Work out the finished part from the listing and answer in its coordinate system (mm). Face numbers are marked on the shaded views. A direction names the side the tool comes from. Round coordinates to 2 decimals unless told otherwise and drop trailing zeros. Loops run counter-clockwise (first coordinate to the right, second up) from the corner with the lowest first, then second, coordinate; pieces in that order, holes last. Notation, with made-up numbers: (-37, 85) -> (-22, 85) arc R25 ccw to (-22, 104) -> close; hole circle Ø4 at (-36.5, -26). An arc over 180 degrees is marked (long way). Use one line per item in the form item = value.
```python
from build123d import *

# Parameters (mm, degrees)
F1_DEPTH = 12.7
F3_DEPTH = 38.1
F4_W     = 38.1
F4_H     = 12.7
F5_DEPTH = 50.801
F7_DEPTH = 76.201


with BuildPart() as f1:
    # F0 (on Front) → F1 (new body)
    with BuildSketch(Plane.XZ):
        Polygon((0, 25.4), (0, 0), (76.2, 0), (76.2, 25.4), (50.8, 50.8), (25.4, 50.8), align=None)
    extrude(amount=F1_DEPTH)

    # F2 (on face) → F3 (join)
    with BuildSketch(Plane.XZ.offset(12.7)):
        Polygon((38.1, 50.8), (0, 0), (76.2, 0), align=None)
    extrude(amount=F3_DEPTH)

    # F4 (on face) → F5 (cut, through all)
    with BuildSketch(Plane(origin=(0, 0, 0), x_dir=(-1, 0, 0), z_dir=(0, 1, 0))):
        with Locations((-38.1, 6.35)):
            Rectangle(F4_W, F4_H)
    extrude(amount=-F5_DEPTH, mode=Mode.SUBTRACT)

    # F6 (on face) → F7 (cut, through all)
    with BuildSketch(Plane.YZ.offset(76.2)):
        Polygon((-12.7, 38.1), (-12.7, 50.8), (-50.8, 50.8), (-50.8, 0), align=None)
    extrude(amount=-F7_DEPTH, mode=Mode.SUBTRACT)


solid = f1.part
```
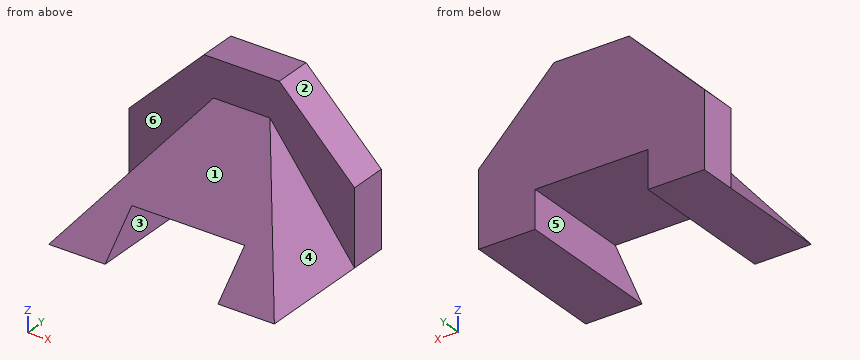
(1) Find section C-C, the plane x = 66. Write down the section's boundary in (y, z).
Completed:
outline = (-50.8, 0) -> (0, 0) -> (0, 35.6) -> (-12.7, 35.6) -> (-12.7, 13.6) -> (-37.2, 13.6) -> close
(2) Find section A-A, the plane y = -41. Write down the section's boundary in (x, z), then the cut area to 3 significant figures.
Completed:
outline = (0, 0) -> (19.05, 0) -> (19.05, 9.8) -> (7.35, 9.8) -> close; (57.15, 0) -> (76.2, 0) -> (68.85, 9.8) -> (57.15, 9.8) -> close
area = 301 mm2
(3) For the marked faces 4, 5 and 6, determine the directions among +Z, -Z, +X, -X, +Y, -Y from which every point of the face is accessible in a straight line to the end or side of a thin tool.
Completed:
face_4 = +Z, +X, -Y
face_5 = -Z, +Y, -Y
face_6 = +Z, -Y
(4) Find section B-B, the plane y = -29. Write down the section's boundary in (x, z), then the cut area to 3 significant figures.
Completed:
outline = (0, 0) -> (19.05, 0) -> (19.05, 12.7) -> (57.15, 12.7) -> (57.15, 0) -> (76.2, 0) -> (59.85, 21.8) -> (16.35, 21.8) -> close
area = 821 mm2
(5) For a pull along X with two mould halves and no side action, classify the marked faces 1, 2 and 3 as +X half, -X half, draft (parallel to the pull), parting line (faces both ways), or undercut.
Completed:
face_1 = draft
face_2 = +X half
face_3 = undercut
(6) Find section D-D, the plane z = 22.5. Write down the section's boundary in (x, y) (3 decimals).
Completed:
outline = (0, -12.7) -> (16.875, -12.7) -> (16.875, -28.3) -> (59.325, -28.3) -> (59.325, -12.7) -> (76.2, -12.7) -> (76.2, 0) -> (0, 0) -> close
(7) Given P1, Ø6, axis at x = 16, y = -25.5, coming from the +Z side; P2, Ø6, axis at y = -45.5, z = 10.5, coming from the -X side; P3, Ø1, axis at x = 27.5, y = -36.5, coming from the +Z side; P4, Ø12, axis at y = -11, z = 35, coming from the -X side, each flat-ended and moving along its own axis, determine where each tip first touches the part or whether it passes through.
Completed:
P1 = 25.33
P2 = through
P3 = 14.8
P4 = 3.6
(8) Consider L1, parallel to X at y = -10.5, z = 5; L2, parallel to Y at x = 73, z = 21; L3, parallel to Z at x = 21.5, y = -10.5. Determine where each line is inside the solid, lowest interval first.
Completed:
L1 = 0 to 19.05, 57.15 to 76.2
L2 = -12.7 to 0
L3 = 12.7 to 46.9
